```python
from build123d import *

# Parameters (mm, degrees)
SKETCH_1_W = 1.4
SKETCH_1_H = 2


with BuildPart() as part:
    # Эскиз1 → Повернуть8 (revolve)
    with BuildSketch(Plane.XY, mode=Mode.PRIVATE) as revolve_8_sk:
        with BuildLine():
            Line((28.8, 4.8), (10.2, 4.8))
            Line((10.2, 4.8), (10.2, 0))
            Line((10.2, 0), (32, 0))
            Line((32, 0), (32, 8))
            ThreePointArc((32, 8), (29.7372583, 7.0627417), (28.8, 4.8))
        make_face()
        with BuildLine():
            ThreePointArc((10.2, 4.8), (9.2627417, 7.0627417), (7, 8))
            Line((7, 8), (7, 0))
            Line((7, 0), (10.2, 0))
            Line((10.2, 0), (10.2, 4.8))
        make_face()
        with BuildLine():
            Line((0, 10), (0, 0))
            Line((0, 0), (1, 0))
            Line((1, 0), (1, 5.25))
            Line((1, 5.25), (3.5, 5.25))
            Line((3.5, 5.25), (3.5, 0))
            Line((3.5, 0), (7, 0))
            Line((7, 0), (7, 8))
            ThreePointArc((7, 8), (6.414213562, 9.414213562), (5, 10))
            Line((5, 10), (0, 10))
        make_face()
        Polygon((32, 8), (32, 0), (35, 0), (35, 2), (35, 8), align=None)
        with Locations((35.7, 1)):
            Rectangle(SKETCH_1_W, SKETCH_1_H)
        with BuildLine():
            Line((36.4, 2), (36.4, 0))
            Line((36.4, 0), (52.145966692, 0))
            ThreePointArc((52.145966692, 0), (45.154001032, 7.93623757), (36.4, 2))
        make_face()
    revolve(revolve_8_sk.sketch.rotate(Axis((0, 0, 0), (1, 0, 0)), 90), axis=Axis((0, 0, 0), (1, 0, 0)))


solid = part.part
```
CAD build for the part. Positions are in the model's coordinates, mm. A direction names the side the tool comes from. Round coordinates to 2 decimals unless told otherwise and drop trailing zeros. Loops run counter-clockwise (first coordinate to the right, second up) from the corner with the lowest first, then second, coordinate; pieces in that order, holes last. Notation, with made-up numbers: M -5,11.5 L 8,11.5 A17 ccw 8,22.5 Z; hole C 59,83.5 d4. An arc over 180 degrees is marked long. Use a Markdown table: item, result. Add a question column.
(1) Drill centre lines: line 1 (Y direction, x = 1.8, z = 0); line 2 (X direction, y = -5.25, z = -1); line 3 (X direction, y = 3, z = 0.5). Where is each one in solid material? Low to high.
(2) Cut at D-D (x = 25). Give the cut face in (y, z).
(3) Pull direction Y, two halves, no side cores. Call faces 3 (the face through (2.3, -1.6, 5)), 4 (the face through (33.48, 7.81, -1.73)), 5 (the face through (0, 0, 0)): +Y half, -Y half, draft (parallel to the pull), parting line (faces both ways), or undercut.
(4) Cut at C-C (y = -7). State how many separate pieces and enclosed holes the cut face has, and give its area (3 significant figures).
(5) Flat gauge pins, fed straight in: pin 1 (8 mm diameter, centred on y = 2.5, z = -5, fed in from +X); pin 2 (12 mm diameter, centred on y = 5, z = -6.5, fed in from +X); pin 3 (1.5 mm diameter, centred on y = 4, z = -6, fed in from +X); pin 4 (5 mm diameter, centred on x = 21.5, z = -7.5, fed in from +Y). Where does each tip first touch, or does it go through?
(6) Which spindle directions (+Z, -Z, +X, -X, +Y, -Y) get a long thin tool onto all of the face, cutting with end or side? Do faces 1 (the face through (2, 0, -10)), 2 (the face through (36, 2, 0)). Say none if no direction does.
(7) Cut at A-A (z = 0). Give the cut face in (x, y).
Geometry says:
| question | item | result |
|---|---|---|
| 1 | line 1 | y = -10 to -5.25, 5.25 to 10 |
| 1 | line 2 | x = 0 to 10.15, 28.85 to 35, 38.19 to 50.1 |
| 1 | line 3 | x = 0 to 1, 3.5 to 35, 36.75 to 51.55 |
| 2 | outline | C 0,0 d9.6 |
| 3 | face 3 | undercut |
| 3 | face 4 | parting line |
| 3 | face 5 | draft |
| 4 | separate pieces | 3 |
| 4 | enclosed holes | 0 |
| 4 | area | 196 mm² |
| 5 | pin 1 | stops at x = 51.99 |
| 5 | pin 2 | stops at x = 51.84 |
| 5 | pin 3 | stops at x = 48.86 |
| 5 | pin 4 | passes through |
| 6 | face 1 | +X, -X |
| 6 | face 2 | none |
| 7 | outline | M 0,-10 L 5,-10 A2 ccw 7,-8 A3.2 ccw 10.2,-4.8 L 28.8,-4.8 A3.2 ccw 32,-8 L 35,-8 L 35,-2 L 36.4,-2 A8 ccw long 36.4,2 L 35,2 L 35,8 L 32,8 A3.2 ccw 28.8,4.8 L 10.2,4.8 A3.2 ccw 7,8 A2 ccw 5,10 L 0,10 Z; hole M 1,-5.25 L 3.5,-5.25 L 3.5,5.25 L 1,5.25 Z |
